The listing builds one solid part. Answer for the finished solid, in the listing's coordinates (mm). Face numbers are marked on the shaded views. Coordinates: 2 decimals unless noted, no trailing zeros. Order: outer loops, then holes, each group sorted by start corner. A loop starts at its lowest first (then second) coordinate and runs counter-clockwise, first axis right, second up. Notation, with made-up numbers: (-37, 87) - (-31, 87) arc R25 cw to (-31, 106) - close; hole circle Ø3 at (31, -8). An arc over 180 degrees is marked (long way). Use a Markdown table: item, result. Add a question column.
Item 1: The mould has two halves that part along X. Classify the marked faces 1, 2 and 3: released by +X, released by -X, zero draft, split by the parting line, or undercut.
Item 2: The part is cut by section A-A, the plane x = 34. Give the vertices of the cut face in (y, z) (3 decimals).
Item 3: The part is cut by section C-C, the plane y = -15. Give the vertices of the cut face in (x, z).
Item 4: Find the intervals of material crossed by line 1 along Z through (x, y) = (14.5, 3); line 2 along X through (y, z) = (-2, 16.5); line 3 along Y through (x, z) = (13, 17), in increasing order.
Item 5: The part is cut by section B-B, the plane z = 14.75. Give the vertices of the cut face in (x, y) (3 decimals).
Item 6: Flat-ended cylindrical pins translate along their axes: P1, Ø12, axis at x = 11, y = -0.5, coming from the +Z side; P2, Ø20, axis at x = 10, y = -6, coming from the -Z side; P3, Ø4, axis at x = 6.5, z = 16, coming from the -Y side. Find the tip coordinate at first contact, or state that the pin passes through.
Item 7: The part is cut by section D-D, the plane z = 20. Give the vertices of the cut face in (x, y) (3 decimals).
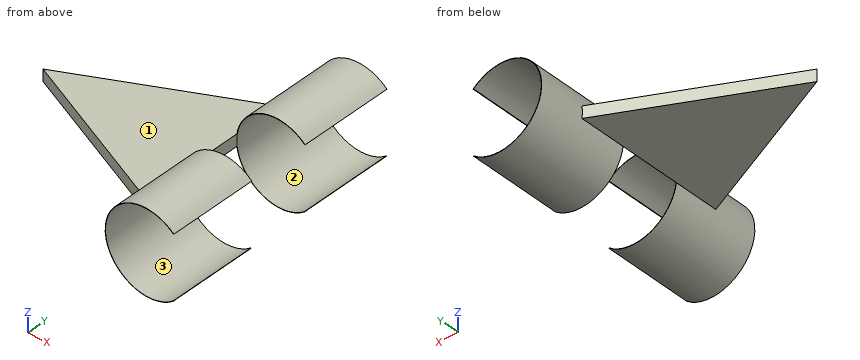
from build123d import *

# Parameters (mm, degrees)
F1_R      = 7.05
F1_R_2    = 7
F2_DEPTH  = 15.357
F4_R      = 7.05
F4_R_2    = 7
F5_DEPTH  = 14.641
F8_DEPTH  = 1
F10_W     = 43.367601
F10_H     = 10.774177
F11_DEPTH = 25


with BuildPart() as f2:
    # F1 (on offset) → F2 (new body)
    with BuildSketch(Plane.XZ.offset(-4.645)):
        with Locations((34, 17.05)):
            Circle(F1_R)
        with Locations((34, 17.05)):
            Circle(F1_R_2, mode=Mode.SUBTRACT)
    extrude(amount=-F2_DEPTH)



with BuildPart() as f5:
    # F4 (on offset) → F5 (new body)
    with BuildSketch(Plane.XZ.offset(5.359)):
        with Locations((34, 17.05)):
            Circle(F4_R)
        with Locations((34, 17.05)):
            Circle(F4_R_2, mode=Mode.SUBTRACT)
    extrude(amount=F5_DEPTH)


with BuildPart() as f2_1:
    add(f2.part)

    add(f5.part)  # F8 merges F5
    # F7 (on offset) → F8 (join, symmetric)
    with BuildSketch(Plane.XY.offset(17.05)):
        Polygon((27, -12.721453), (27, 12.37814), (0, -1.858111), align=None)
    extrude(amount=F8_DEPTH, both=True)

    # F10 (on offset) → F11 (cut)
    with BuildSketch(Plane.YZ.offset(38.5)):
        with Locations((0.986395, 17.003338)):
            Rectangle(F10_W, F10_H)
    extrude(amount=F11_DEPTH, mode=Mode.SUBTRACT)


solid = f2_1.part
Solution:
| question | item | result |
|---|---|---|
| 1 | face 1 | zero draft |
| 1 | face 2 | undercut |
| 1 | face 3 | undercut |
| 2 | outline | (-20, 10) - (-5.359, 10) - (-5.359, 10.05) - (-20, 10.05) - close; (-20, 24.05) - (-5.359, 24.05) - (-5.359, 24.1) - (-20, 24.1) - close; (4.645, 10) - (20.002, 10) - (20.002, 10.05) - (4.645, 10.05) - close; (4.645, 24.05) - (20.002, 24.05) - (20.002, 24.1) - (4.645, 24.1) - close |
| 3 | outline | (38.5, 11.62) - (38.5, 11.69) arc R7 cw (long way) to (38.53, 22.39) - (38.6, 22.39) arc R7.05 ccw (long way) to start |
| 4 | line 1 | z = 16.05 to 18.05 |
| 4 | line 2 | x = 0.35 to 27 |
| 4 | line 3 | y = -7.09 to 5 |
| 5 | outline | (27.336, -20) - (27.389, -20) - (27.389, -5.359) - (27.336, -5.359) - close; (27.336, 4.645) - (27.389, 4.645) - (27.389, 20.002) - (27.336, 20.002) - close |
| 6 | P1 | stops at z = 18.05 |
| 6 | P2 | stops at z = 16.05 |
| 6 | P3 | stops at y = -5.28 |
| 7 | outline | (27.597, -20) - (27.652, -20) - (27.652, -5.359) - (27.597, -5.359) - close; (27.597, 4.645) - (27.652, 4.645) - (27.652, 20.002) - (27.597, 20.002) - close |
